Could you check a few things on this model? Use its own coordinates, in mm. Face numbers are marked on the shaded views. A direction names the side the tool comes from. Round coordinates to 2 decimals unless told otherwise and drop trailing zeros. Order: outer loops, then holes, each group sorted by start corner. A loop starts at its lowest first (then second) coordinate and runs counter-clockwise, first axis right, second up. Notation, with made-up numbers: (-19.75, 42) - (19.25, 42) arc R23 cw to (19.25, 77) - close; hole circle Ø2 at (52.5, 25.5). An arc over 180 degrees is marked (long way). Use one line per item in the form item = value.
from build123d import *

# Parameters (mm, degrees)
F1_DEPTH = 4


# Not quite as in the source:
# - a feature names something its author has since deleted; it is built from what else it names


with BuildPart() as f1:
    # F0 (on Top) → F1 (new body)
    with BuildSketch(Plane.XY):
        with BuildLine():
            ThreePointArc((-20.4431954222, -12.9176859982), (-15.6048127823, -13.347574962), (-11.2276054917, -15.453473209))
            ThreePointArc((-11.2276054917, -15.453473209), (-7.8721458006, -18.9656863791), (-5.9681546392, -23.4344187216))
            Line((-5.9681546392, -23.4344187216), (0, -19.0983005625))
            Line((0, -19.0983005625), (6.2352903352, -23.6285041655))
            ThreePointArc((6.2352903352, -23.6285041655), (8.0892727444, -19.1867619995), (11.4055803613, -15.6984346018))
            ThreePointArc((11.4055803613, -15.6984346018), (15.747972276, -13.6223910806), (20.5452321785, -13.2317228431))
            Line((20.5452321785, -13.2317228431), (18.1635632001, -5.9016994375))
            Line((18.1635632001, -5.9016994375), (24.3988535354, -1.3714958345))
            ThreePointArc((24.3988535354, -1.3714958345), (18.4546166861, 5.9962684477), (18.9329421283, 15.4508497187))
            Line((18.9329421283, 15.4508497187), (15.537885835, 15.4508497187))
            Line((15.537885835, 15.4508497187), (11.2256994145, 15.4508497187))
            Line((11.2256994145, 15.4508497187), (8.8582927724, 22.7369781668))
            ThreePointArc((8.8582927724, 22.7369781668), (4.7280277023, 20.2947827391), (0, 19.4767594488))
            ThreePointArc((0, 19.4767594488), (-4.7153721091, 20.3911605121), (-8.7986573229, 22.920517208))
            Line((-8.7986573229, 22.920517208), (-11.2256994145, 15.4508497187))
            Line((-11.2256994145, 15.4508497187), (-18.184390629, 15.4508497187))
            ThreePointArc((-18.184390629, 15.4508497187), (-17.4535891597, 12.9689141671), (-17.2070021976, 10.3934006765))
            ThreePointArc((-17.2070021976, 10.3934006765), (-17.4045597984, 8.086010366), (-17.9914818172, 5.8457868068))
            ThreePointArc((-17.9914818172, 5.8457868068), (-20.4374126709, 1.6036270131), (-24.2294812931, -1.4945519715))
            Line((-24.2294812931, -1.4945519715), (-18.1635632001, -5.9016994375))
            Line((-18.1635632001, -5.9016994375), (-20.4431954222, -12.9176859982))
        make_face()
        with BuildLine():
            ThreePointArc((14.5987175251, 4.7434108637), (15.1610160281, 2.4012690384), (15.35, 0))
            ThreePointArc((15.35, 0), (15.1610160281, -2.4012690384), (14.5987175251, -4.7434108637))
            ThreePointArc((14.5987175251, -4.7434108637), (12.4184108637, -9.0225036227), (9.0225036227, -12.4184108637))
            ThreePointArc((9.0225036227, -12.4184108637), (4.7434108637, -14.5987175251), (0, -15.35))
            ThreePointArc((0, -15.35), (-4.7434108637, -14.5987175251), (-9.0225036227, -12.4184108637))
            ThreePointArc((-9.0225036227, -12.4184108637), (-12.4184108637, -9.0225036227), (-14.5987175251, -4.7434108637))
            ThreePointArc((-14.5987175251, -4.7434108637), (-15.35, 0), (-14.5987175251, 4.7434108637))
            ThreePointArc((-14.5987175251, 4.7434108637), (-12.4184108637, 9.0225036227), (-9.0225036227, 12.4184108637))
            ThreePointArc((-9.0225036227, 12.4184108637), (-4.7434108637, 14.5987175251), (0, 15.35))
            ThreePointArc((0, 15.35), (4.7434108637, 14.5987175251), (9.0225036227, 12.4184108637))
            ThreePointArc((9.0225036227, 12.4184108637), (12.4184108637, 9.0225036227), (14.5987175251, 4.7434108637))
        make_face(mode=Mode.SUBTRACT)
    extrude(amount=F1_DEPTH)


solid = f1.part
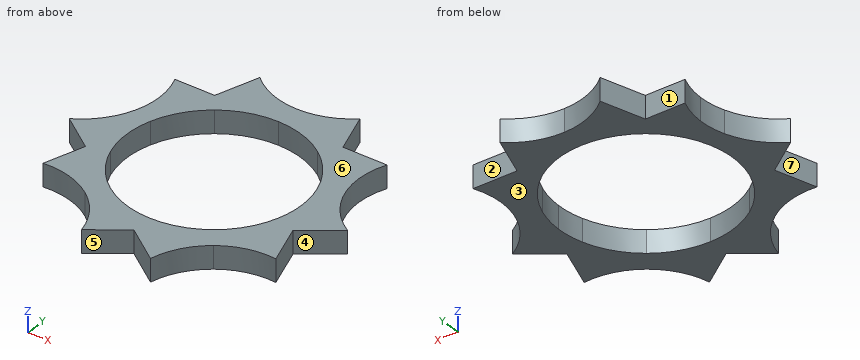
Item 1: If we mould it in two halves opening along Y, with no side actions, what happens to the marked faces 4, 5, 6 and 7? For each: released by +Y, released by -Y, zero draft, split by the parting line, or undercut.
Found:
face_4 = undercut
face_5 = released by -Y
face_6 = zero draft
face_7 = undercut
Item 2: For the marked faces 1, 2 and 3, which set-ups out of +Z, -Z, +X, -X, +Y, -Y let a thin tool reach every point of the face, with its end or its side?
Found:
face_1 = +Z, -Z, -X, +Y
face_2 = +Z, -Z, +X, +Y
face_3 = -Z, +X, -X, +Y, -Y
Item 3: Imagine slicing it at A-A on z = 2.45. Please give me the cut outline in (x, y), plus the area to 3 significant figures.
Found:
outline = (-24.23, -1.49) - (-18.16, -5.9) - (-20.44, -12.92) arc R13.57 cw to (-5.97, -23.43) - (0, -19.1) - (6.24, -23.63) arc R13.27 cw to (20.55, -13.23) - (18.16, -5.9) - (24.4, -1.37) arc R13.27 cw to (18.93, 15.45) - (11.23, 15.45) - (8.86, 22.74) arc R13.3 cw to (-8.8, 22.92) - (-11.23, 15.45) - (-18.18, 15.45) arc R13.57 cw to start; hole circle Ø30.7 at (0, 0)
area = 644 mm2
Item 4: Imagine slicing it at D-D on x = -16. Please give me the cut outline in (y, z), plus the area to 3 significant figures.
Found:
outline = (-13.25, 0) - (15.45, 0) - (15.45, 4) - (-13.25, 4) - close
area = 115 mm2
Item 5: I need wall thicknesses on L1, parallel to Y at x = -16, z = 3.8; L2, parallel to X at y = -3, z = 2.4; L3, parallel to Y at x = -3, z = 2.45. Which ranges of each line are inside material? Lowest first, please.
Found:
L1 = -13.25 to 15.45
L2 = -22.16 to -15.05, 15.05 to 22.16
L3 = -21.28 to -15.05, 15.05 to 19.85
Item 6: Imagine slicing it at B-B on y = -10. Please give me the cut outline in (x, z), plus the area to 3 significant figures.
Found:
outline = (-19.5, 0) - (-11.65, 0) - (-11.65, 4) - (-19.5, 4) - close; (11.65, 0) - (19.5, 0) - (19.5, 4) - (11.65, 4) - close
area = 62.8 mm2
Item 7: Imagine slicing it at C-C on x = 1. Please give me the cut outline in (y, z), plus the area to 3 significant figures.
Found:
outline = (-19.82, 0) - (-15.32, 0) - (-15.32, 4) - (-19.82, 4) - close; (15.32, 0) - (19.5, 0) - (19.5, 4) - (15.32, 4) - close
area = 34.8 mm2
Item 8: Will these pins go through, and if not, where does the flat tip stop? P1, Ø1, axis at x = 0.5, y = 15.5, coming from the -Z side; P2, Ø2, axis at x = -16, z = 2.5, coming from the +Y side; P3, Ø1.5, axis at y = -5, z = 1, coming from the -X side.
Found:
P1 = 0
P2 = 15.45
P3 = -20.44
